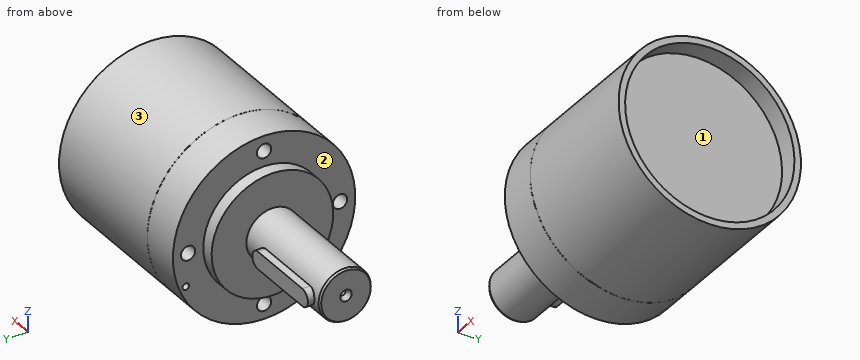
```python
from build123d import *

# Parameters (mm, degrees)
SKETCH2_R                              = 14
BOSS_EXTRUDE1_DEPTH                    = 3
SKETCH3_R                              = 6
BOSS_EXTRUDE2_DEPTH                    = 26.5
BOSS_EXTRUDE4_REACH                    = 56.169
BOSS_EXTRUDE4_END_RADIUS               = 6
M36_CLEARANCE_HOLE1_D                  = 39
M36_CLEARANCE_HOLE1_DEPTH              = 4.45
F_1_5_1_5_DIAMETER_HOLE1_D             = 1.5
F_1_5_1_5_DIAMETER_HOLE1_DEPTH         = 2
F_1_5_1_5_DIAMETER_HOLE1_TIP           = 0.450645464
F_3_3_3_3_DIAMETER_HOLE1_D             = 3.3
F_3_3_3_3_DIAMETER_HOLE1_DEPTH         = 6
F_3_3_3_3_DIAMETER_HOLE1_TIP           = 0.991420021
F_1_25_1_25_DIAMETER_HOLE1_D           = 1.25
F_1_25_1_25_DIAMETER_HOLE1_DEPTH       = 1.939156082
F_1_25_1_25_DIAMETER_HOLE1_CSINK_D     = 2.65
F_1_25_1_25_DIAMETER_HOLE1_CSINK_ANGLE = 60
F_1_25_1_25_DIAMETER_HOLE1_TIP         = 0.360843918
CHAMFER1_SIZE                          = 0.288675135
CHAMFER1_SIZE2                         = 0.5


with BuildPart() as part:
    # Sketch1 → Revolve1 (revolve)
    with BuildSketch(Plane.XY, mode=Mode.PRIVATE) as revolve1_sk:
        with BuildLine():
            Line((0, 21), (0, 0))
            Line((0, 0), (41, 0))
            Line((41, 0), (41, 21))
            Line((41, 21), (9.25, 21))
            ThreePointArc((9.25, 21), (9.2, 20.98660254), (9.15, 21))
            Line((9.15, 21), (0, 21))
        make_face()
    revolve(revolve1_sk.sketch.rotate(Axis((0, 0, 0), (1, 0, 0)), 270), axis=Axis((0, 0, 0), (1, 0, 0)))

    # Sketch2 → Boss-Extrude1 (add)
    with BuildSketch(Plane.ZY):
        Circle(SKETCH2_R)
    extrude(amount=BOSS_EXTRUDE1_DEPTH)

    # Sketch3 → Boss-Extrude2 (add)
    with BuildSketch(Plane.ZY.offset(3)):
        Circle(SKETCH3_R)
    extrude(amount=BOSS_EXTRUDE2_DEPTH)

    # Boss-Extrude4: up to this cylinder (the profile starts outside it)
    boss_extrude4_end = Plane(origin=(-17.5, 0, 0), z_dir=(1, 0, 0)) * Cylinder(BOSS_EXTRUDE4_END_RADIUS, 125.338, mode=Mode.PRIVATE)
    # Sketch5 → Boss-Extrude4 (add, up to the surface)
    with BuildSketch(Plane(origin=(0, 7.5, 0), x_dir=(1, 0, 0), z_dir=(0, 1, 0)), mode=Mode.PRIVATE) as boss_extrude4_sk1:
        with BuildLine():
            Line((-9.5, 2), (-25.5, 2))
            ThreePointArc((-25.5, 2), (-27.5, 0), (-25.5, -2))
            Line((-25.5, -2), (-9.5, -2))
            ThreePointArc((-9.5, -2), (-7.5, 0), (-9.5, 2))
        make_face()
    boss_extrude4_tool1 = extrude(boss_extrude4_sk1.sketch, amount=-BOSS_EXTRUDE4_REACH, mode=Mode.PRIVATE) - boss_extrude4_end
    add(boss_extrude4_tool1.solids().sort_by_distance((-17.5, 7.5, 0))[0])

    # M36 Clearance Hole1
    with Locations(Plane(origin=(41, 0, 0), x_dir=(0, 0, -1), z_dir=(1, 0, 0))):
        with Locations((0, 0)):
            Hole(M36_CLEARANCE_HOLE1_D / 2, depth=M36_CLEARANCE_HOLE1_DEPTH)

    # Ø1.5 (1.5) Diameter Hole1
    with Locations(Plane.ZY):
        with Locations((-7.462326931, 18.015650884)):
            Hole(F_1_5_1_5_DIAMETER_HOLE1_D / 2, depth=F_1_5_1_5_DIAMETER_HOLE1_DEPTH)
            with Locations((0, 0, -(F_1_5_1_5_DIAMETER_HOLE1_DEPTH + F_1_5_1_5_DIAMETER_HOLE1_TIP / 2))):  # 118° drill point
                Cone(0, F_1_5_1_5_DIAMETER_HOLE1_D / 2, F_1_5_1_5_DIAMETER_HOLE1_TIP, mode=Mode.SUBTRACT)

    # Ø3.3 (3.3) Diameter Hole1
    with Locations(Plane.ZY):
        with Locations((3.0543e-05, 17.5), (17.5, -3.0543e-05), (-3.0543e-05, -17.5), (-17.5, 3.0543e-05)):
            Hole(F_3_3_3_3_DIAMETER_HOLE1_D / 2, depth=F_3_3_3_3_DIAMETER_HOLE1_DEPTH)
            with Locations((0, 0, -(F_3_3_3_3_DIAMETER_HOLE1_DEPTH + F_3_3_3_3_DIAMETER_HOLE1_TIP / 2))):  # 118° drill point
                Cone(0, F_3_3_3_3_DIAMETER_HOLE1_D / 2, F_3_3_3_3_DIAMETER_HOLE1_TIP, mode=Mode.SUBTRACT)

    # Ø1.25 (1.25) Diameter Hole1
    with Locations(Plane.ZY.offset(29.5)):
        with Locations((0, 0)):
            CounterSinkHole(F_1_25_1_25_DIAMETER_HOLE1_D / 2, F_1_25_1_25_DIAMETER_HOLE1_CSINK_D / 2, depth=F_1_25_1_25_DIAMETER_HOLE1_DEPTH, counter_sink_angle=F_1_25_1_25_DIAMETER_HOLE1_CSINK_ANGLE)
            with Locations((0, 0, -(F_1_25_1_25_DIAMETER_HOLE1_DEPTH + F_1_25_1_25_DIAMETER_HOLE1_TIP / 2))):  # 120° drill point
                Cone(0, F_1_25_1_25_DIAMETER_HOLE1_D / 2, F_1_25_1_25_DIAMETER_HOLE1_TIP, mode=Mode.SUBTRACT)

    # Chamfer1
    chamfer1_edges = [part.edges().sort_by_distance(p)[0] for p in [
        (-29.5, 0, -6),
    ]]
    chamfer1_side = [part.faces().sort_by_distance(p)[0] for p in [
        (-29.5, 0, -5.830294373),
    ]]
    chamfer(chamfer1_edges, length=CHAMFER1_SIZE, length2=CHAMFER1_SIZE2, reference=chamfer1_side[0])


solid = part.part
```
Check sheet for the modelled part. Datum: model origin and axes. Units: mm. Face numbers are marked on the shaded views. Give positions to 0.01 mm unless a question says otherwise; leave off trailing zeros. Loops run counter-clockwise (first coordinate to the right, second up) from the corner with the lowest first, then second, coordinate; pieces in that order, holes last. Notation, with made-up numbers: (75, 50.25) - (95, 50.25) arc R34 cw to (95, 82.25) - close; hole circle Ø2 at (36, -8.75). An arc over 180 degrees is marked (long way). One line per question, with ' | ' between items. Start each with the question number.
1. Material ranges on line 1 along Y through (x, z) = (39.6, 0); line 2 along X through (y, z) = (-7, -8); line 3 along Y through (x, z) = (21, 0.5), recorded low to high. Write a range as [from, to].
2. Gauge pin test, flat ends, axial feed: pin 1 Ø4 at (y, z) = (0, 17.5) entering from -X; pin 2 Ø8 at (x, z) = (29, 16) entering from -Y; pin 3 Ø1.5 at (x, y) = (-20.5, 6.5) entering from -Z. Record the tip position at first contact, or that the pin passes through.
3. Draft check along Z on the marked faces 1, 2 and 3. Enter one of: released by +Z, released by -Z, zero draft, split by the parting line, or undercut.
4. Cross-section at B-B, the plane x = 24.5. Enter the section's corners in (y, z), plus the area to 3 significant figures.
5. Cross-section at A-A, the plane x = -17.5. Enter the section's corners in (y, z), plus the area to 3 significant figures.
Check result:
1) line 1: y = [-21, -19.5], [19.5, 21] | line 2: x = [-3, 36.55] | line 3: y = [-20.99, 20.99]
2) pin 1: stops at x = 0 | pin 2: stops at y = -17.23 | pin 3: stops at z = -2
3) face 1: undercut | face 2: zero draft | face 3: split by the parting line
4) outline: circle Ø42 at (0, 0) | area: 1,390 mm2
5) outline: (5.66, -2) - (7.5, -2) - (7.5, 2) - (5.66, 2) arc R6 ccw (long way) to start | area: 120 mm2
